Design review of the part built by this model. Coordinates are the model's own, in mm. Face numbers are marked on the shaded views. A direction names the side the tool comes from. Round coordinates to 2 decimals unless told otherwise and drop trailing zeros. Write each loop counter-clockwise with the first axis right and the second up, starting at its lowest first coordinate (ties: lowest second). Pieces come first, ordered by that corner, then holes. Notation, with made-up numbers: M 43,79.5 L 79,79.5 A24 ccw 79,117.5 Z; hole C 30,-12.75 d7. An arc over 180 degrees is marked long. One line per question, with ' | ' between items. Start each with the question number.
Item 1: For L1, parallel to Z at x = -36.5, y = -27.5; L2, parallel to X at y = -3.5, z = -1.5; L3, parallel to Z at x = -28.5, y = -25.5, list the stretches that pass through material, from the lowest coordinate up.
Item 2: Add section A-A, the plane z = -1.9. State the section outline as (x, y) points, and give its area (3 significant figures).
Item 3: Add section C-C, the plane y = -29. State the section outline as (x, z) points, and give its area (3 significant figures).
Item 4: Insertion check: pin 1 Ø4.5 at (x, y) = (-45.99, -3.19) entering from +Z; pin 2 Ø2 at (x, y) = (-55.99, -10.69) entering from -Z; pin 3 Ø7.5 at (x, y) = (-56.5, -3.5) entering from +Z. Each pin has a flat end and moves straight along its axis. Give the tip position at first contact, or say it passes through.
Item 5: Machinability: for the marked faces 1, 2 and 3, which of the approach directions +Z, -Z, +X, -X, +Y, -Y give a long, thin tool a straight path to every point of the face, cutting with its end or side? Answer none if there is none.
Item 6: Add section D-D, the plane z = 1.25. State the section outline as (x, y) points.
Item 7: Add section B-B, the plane x = -58.5. State the section outline as (y, z) points.
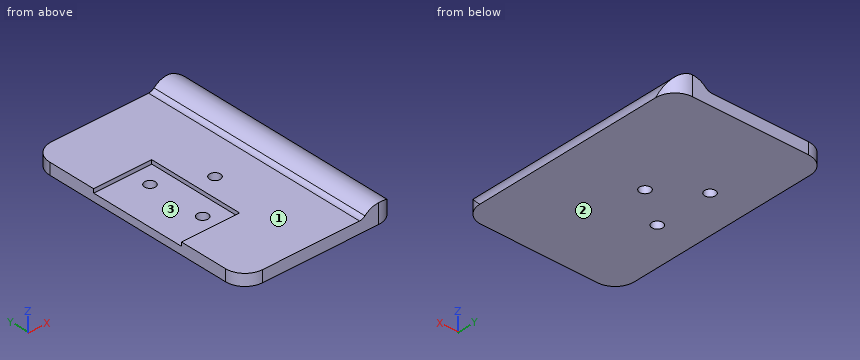
```python
from build123d import *

# Parameters (mm, degrees)
SKETCH1_W                  = 40
SKETCH1_H                  = 60
BOSS_EXTRUDE1_DEPTH        = 3
SKETCH2_W                  = 15
SKETCH2_H                  = 25
CUT_EXTRUDE1_DEPTH         = 1
F_2_8_2_8_DIAMETER_HOLE1_D = 2.8
F_2_8_2_8_DIAMETER_HOLE2_D = 2.8
FILLET1_R                  = 5
BOSS_EXTRUDE2_DEPTH        = 36.5
CUT_EXTRUDE3_DEPTH         = 126
CUT_EXTRUDE4_START         = -126
SKETCH11_W                 = 58.073467033
SKETCH11_H                 = 92.384025597
CUT_EXTRUDE4_DEPTH         = 126
FILLET2_R                  = 2


with BuildPart() as part:
    # Sketch1 → Boss-Extrude1 (new body)
    with BuildSketch(Plane(origin=(0, 0, -3), x_dir=(-1, 0, 0), z_dir=(0, 0, -1))):
        with Locations((45.9850693, -3.193565597)):
            Rectangle(SKETCH1_W, SKETCH1_H)
    extrude(amount=-BOSS_EXTRUDE1_DEPTH)

    # Sketch2 → Cut-Extrude1 (cut)
    with BuildSketch(Plane.XY):
        with Locations((-58.4850693, -3.193565597)):
            Rectangle(SKETCH2_W, SKETCH2_H)
    extrude(amount=-CUT_EXTRUDE1_DEPTH, mode=Mode.SUBTRACT)

    # 2.8 _2.8_ Diameter Hole1 (through all)
    with Locations(Plane.XY):
        with Locations((-45.9850693, -3.193565597)):
            Hole(F_2_8_2_8_DIAMETER_HOLE1_D / 2)

    # 2.8 _2.8_ Diameter Hole2 (through all)
    with Locations(Plane.XY.offset(-1)):
        with Locations((-55.9850693, 4.306434403), (-55.9850693, -10.693565597)):
            Hole(F_2_8_2_8_DIAMETER_HOLE2_D / 2)

    # Fillet1
    fillet1_edges = [part.edges().sort_by_distance(p)[0] for p in [
        (-65.9850693, -33.193565597, -1.5),
        (-25.9850693, -33.193565597, -1.5),
        (-25.9850693, 26.806434403, -1.5),
        (-65.9850693, 26.806434403, -1.5),
    ]]
    fillet(fillet1_edges, radius=FILLET1_R)

    # Sketch8 → Boss-Extrude2 (add, symmetric)
    with BuildSketch(Plane(origin=(0, 0, 0), x_dir=(1, 0, 0), z_dir=(0, 1, 0))):
        with BuildLine():
            Line((-35.9850693, 3), (-25.9850693, 3))
            ThreePointArc((-25.9850693, 3), (-30.9850693, -2), (-35.9850693, 3))
        make_face()
    extrude(amount=BOSS_EXTRUDE2_DEPTH, both=True)

    # Sketch10 → Cut-Extrude3 (cut)
    with BuildSketch(Plane(origin=(0, 26.806434403, 0), x_dir=(1, 0, 0), z_dir=(0, 1, 0))):
        with BuildLine():
            Line((-26.9850693, 0), (-25.9850693, 0))
            Line((-25.9850693, 0), (-25.9850693, 3))
            ThreePointArc((-25.9850693, 3), (-26.24165281, 1.41886117), (-26.9850693, 0))
        make_face()
    extrude(amount=-CUT_EXTRUDE3_DEPTH, mode=Mode.SUBTRACT)

    # Sketch11 → Cut-Extrude4 (cut)
    with BuildSketch(Plane(origin=(0, 0, -3), x_dir=(-1, 0, 0), z_dir=(0, 0, -1)).offset(CUT_EXTRUDE4_START)):
        with Locations((44.104932563, -0.297791146)):
            Rectangle(SKETCH11_W, SKETCH11_H)
        with BuildLine():
            Line((35.9850693, -33.193565597), (60.9850693, -33.193565597))
            ThreePointArc((60.9850693, -33.193565597), (64.520603206, -31.729099503), (65.9850693, -28.193565597))
            Line((65.9850693, -28.193565597), (65.9850693, 21.806434403))
            ThreePointArc((65.9850693, 21.806434403), (64.520603206, 25.341968309), (60.9850693, 26.806434403))
            Line((60.9850693, 26.806434403), (35.9850693, 26.806434403))
            Line((35.9850693, 26.806434403), (30.9850693, 26.806434403))
            ThreePointArc((30.9850693, 26.806434403), (27.449535394, 25.341968309), (25.9850693, 21.806434403))
            Line((25.9850693, 21.806434403), (25.9850693, -28.193565597))
            ThreePointArc((25.9850693, -28.193565597), (27.449535394, -31.729099503), (30.9850693, -33.193565597))
            Line((30.9850693, -33.193565597), (35.9850693, -33.193565597))
        make_face(mode=Mode.SUBTRACT)
    extrude(amount=CUT_EXTRUDE4_DEPTH, mode=Mode.SUBTRACT)

    # Fillet2
    fillet2_edges = [part.edges().sort_by_distance(p)[0] for p in [
        (-34.9850693, -3.193565597, 0),
    ]]
    fillet(fillet2_edges, radius=FILLET2_R)


solid = part.part
```
Computed values:
1) L1: z = -3 to 0 | L2: x = -65.99 to -47.35, -44.62 to -26.22 | L3: z = -3 to 1.34
2) outline: M -65.99,-28.19 A5 ccw -60.99,-33.19 L -30.99,-33.19 A5 ccw -26.11,-29.29 L -26.11,22.91 A5 ccw -30.99,26.81 L -60.99,26.81 A5 ccw -65.99,21.81 Z; hole C -55.99,-10.69 d2.8; hole C -55.99,4.31 d2.8; hole C -45.99,-3.19 d2.8 | area: 2,350 mm^2
3) outline: M -65.92,-3 L -26.05,-3 L -26.05,-2.19 A5 ccw -34.48,0.57 A2 cw -35.88,0 L -65.92,0 Z | area: 130 mm^2
4) pin 1: stops at z = 0 | pin 2: passes through | pin 3: stops at z = -1
5) face 1: +Z, -X, +Y, -Y | face 2: -Z, +X, -X, +Y, -Y | face 3: +Z, -X
6) outline: M -33.62,-33.19 L -30.99,-33.19 A5 ccw -28.35,-32.44 L -28.35,26.06 A5 ccw -30.99,26.81 L -33.62,26.81 Z
7) outline: M -33.19,-3 L 26.81,-3 L 26.81,0 L 9.31,0 L 9.31,-1 L -15.69,-1 L -15.69,0 L -33.19,0 Z
